```python
from build123d import *

# Parameters (mm, degrees)
SKETCH1_W           = 60
SKETCH1_H           = 50
BOSS_EXTRUDE1_DEPTH = 1
SKETCH2_R           = 0.25
CUT_EXTRUDE1_DEPTH  = 1.5
LPATTERN1_COUNT     = 3
LPATTERN1_PITCH     = 20
SKETCH3_R           = 0.25
CUT_EXTRUDE2_DEPTH  = 1.5
LPATTERN2_COUNT     = 3
LPATTERN2_PITCH     = 20
SKETCH4_R           = 0.5
CUT_EXTRUDE3_DEPTH  = 1.5
SKETCH5_R           = 0.25
CUT_EXTRUDE4_DEPTH  = 1.5
SKETCH6_R           = 0.2
CUT_EXTRUDE5_DEPTH  = 1.5
SKETCH7_R           = 0.25
CUT_EXTRUDE6_DEPTH  = 1.5
LPATTERN3_COUNT     = 7
LPATTERN3_PITCH     = 2.5
SKETCH8_R           = 0.25
CUT_EXTRUDE7_DEPTH  = 1.5
SKETCH9_R           = 0.875
CUT_EXTRUDE8_DEPTH  = 1.5
SKETCH10_R          = 0.5
CUT_EXTRUDE9_DEPTH  = 1.5
SKETCH11_R          = 0.25
CUT_EXTRUDE10_DEPTH = 1.5
SKETCH12_R          = 0.25
CUT_EXTRUDE11_DEPTH = 1.5


with BuildPart() as part:
    # Sketch1 → Boss-Extrude1 (new body)
    with BuildSketch(Plane(origin=(0, 0, 0), x_dir=(1, 0, 0), z_dir=(0, 1, 0))):
        with Locations((30, 25)):
            Rectangle(SKETCH1_W, SKETCH1_H)
    extrude(amount=BOSS_EXTRUDE1_DEPTH)

    # Sketch2 → Cut-Extrude1 (cut)
    with BuildSketch(Plane(origin=(0, 1, 0), x_dir=(1, 0, 0), z_dir=(0, 1, 0))):
        with Locations((10, 7)):
            Circle(SKETCH2_R)
    cut_extrude1 = extrude(amount=-CUT_EXTRUDE1_DEPTH, mode=Mode.SUBTRACT)

    # LPattern1: Cut-Extrude1 ×3
    with Locations(*[(i * LPATTERN1_PITCH, 0, 0) for i in range(1, LPATTERN1_COUNT)]):
        add(cut_extrude1, mode=Mode.SUBTRACT)

    # Sketch3 → Cut-Extrude2 (cut)
    with BuildSketch(Plane(origin=(0, 1, 0), x_dir=(1, 0, 0), z_dir=(0, 1, 0))):
        with Locations((10, 8.5)):
            Circle(SKETCH3_R)
    cut_extrude2 = extrude(amount=-CUT_EXTRUDE2_DEPTH, mode=Mode.SUBTRACT)

    # LPattern2: Cut-Extrude2 ×3
    with Locations(*[(i * LPATTERN2_PITCH, 0, 0) for i in range(1, LPATTERN2_COUNT)]):
        add(cut_extrude2, mode=Mode.SUBTRACT)

    # Sketch4 → Cut-Extrude3 (cut)
    with BuildSketch(Plane(origin=(0, 1, 0), x_dir=(1, 0, 0), z_dir=(0, 1, 0))):
        with Locations((2.5, 20)):
            Circle(SKETCH4_R)
        with Locations((2.5, 25.5)):
            Circle(SKETCH4_R)
    extrude(amount=-CUT_EXTRUDE3_DEPTH, mode=Mode.SUBTRACT)

    # Sketch5 → Cut-Extrude4 (cut)
    with BuildSketch(Plane(origin=(0, 1, 0), x_dir=(1, 0, 0), z_dir=(0, 1, 0))):
        with Locations((10, 20)):
            Circle(SKETCH5_R)
        with Locations((11.25, 22.5)):
            Circle(SKETCH5_R)
        with Locations((8.75, 22.5)):
            Circle(SKETCH5_R)
    extrude(amount=-CUT_EXTRUDE4_DEPTH, mode=Mode.SUBTRACT)

    # Sketch6 → Cut-Extrude5 (cut)
    with BuildSketch(Plane(origin=(0, 1, 0), x_dir=(1, 0, 0), z_dir=(0, 1, 0))):
        with Locations((16.25, 22.5)):
            Circle(SKETCH6_R)
        with Locations((16.25, 28)):
            Circle(SKETCH6_R)
    extrude(amount=-CUT_EXTRUDE5_DEPTH, mode=Mode.SUBTRACT)

    # Sketch7 → Cut-Extrude6 (cut)
    with BuildSketch(Plane(origin=(0, 1, 0), x_dir=(1, 0, 0), z_dir=(0, 1, 0))):
        with Locations((25.25, 28)):
            Circle(SKETCH7_R)
        with Locations((25.25, 20.5)):
            Circle(SKETCH7_R)
    cut_extrude6 = extrude(amount=-CUT_EXTRUDE6_DEPTH, mode=Mode.SUBTRACT)

    # LPattern3: Cut-Extrude6 ×7
    with Locations(*[(i * LPATTERN3_PITCH, 0, 0) for i in range(1, LPATTERN3_COUNT)]):
        add(cut_extrude6, mode=Mode.SUBTRACT)

    # Sketch8 → Cut-Extrude7 (cut)
    with BuildSketch(Plane(origin=(0, 1, 0), x_dir=(1, 0, 0), z_dir=(0, 1, 0))):
        with Locations((50, 35)):
            Circle(SKETCH8_R)
        with Locations((50, 36.5)):
            Circle(SKETCH8_R)
    extrude(amount=-CUT_EXTRUDE7_DEPTH, mode=Mode.SUBTRACT)

    # Sketch9 → Cut-Extrude8 (cut)
    with BuildSketch(Plane(origin=(0, 1, 0), x_dir=(1, 0, 0), z_dir=(0, 1, 0))):
        with Locations((56.5, 46.5)):
            Circle(SKETCH9_R)
        with Locations((3.5, 46.5)):
            Circle(SKETCH9_R)
    extrude(amount=-CUT_EXTRUDE8_DEPTH, mode=Mode.SUBTRACT)

    # Sketch10 → Cut-Extrude9 (cut)
    with BuildSketch(Plane(origin=(0, 1, 0), x_dir=(1, 0, 0), z_dir=(0, 1, 0))):
        with Locations((47, 47)):
            Circle(SKETCH10_R)
        with Locations((41, 47)):
            Circle(SKETCH10_R)
        with Locations((26, 47)):
            Circle(SKETCH10_R)
        with Locations((20, 47)):
            Circle(SKETCH10_R)
    extrude(amount=-CUT_EXTRUDE9_DEPTH, mode=Mode.SUBTRACT)

    # Sketch11 → Cut-Extrude10 (cut)
    with BuildSketch(Plane(origin=(0, 1, 0), x_dir=(1, 0, 0), z_dir=(0, 1, 0))):
        with Locations((47, 43)):
            Circle(SKETCH11_R)
        with Locations((34.5, 43)):
            Circle(SKETCH11_R)
        with Locations((26, 43)):
            Circle(SKETCH11_R)
        with Locations((13.5, 43)):
            Circle(SKETCH11_R)
    extrude(amount=-CUT_EXTRUDE10_DEPTH, mode=Mode.SUBTRACT)

    # Sketch12 → Cut-Extrude11 (cut)
    with BuildSketch(Plane(origin=(0, 1, 0), x_dir=(1, 0, 0), z_dir=(0, 1, 0))):
        with Locations((10, 36.5)):
            Circle(SKETCH12_R)
        with Locations((10, 35)):
            Circle(SKETCH12_R)
    extrude(amount=-CUT_EXTRUDE11_DEPTH, mode=Mode.SUBTRACT)


solid = part.part
```
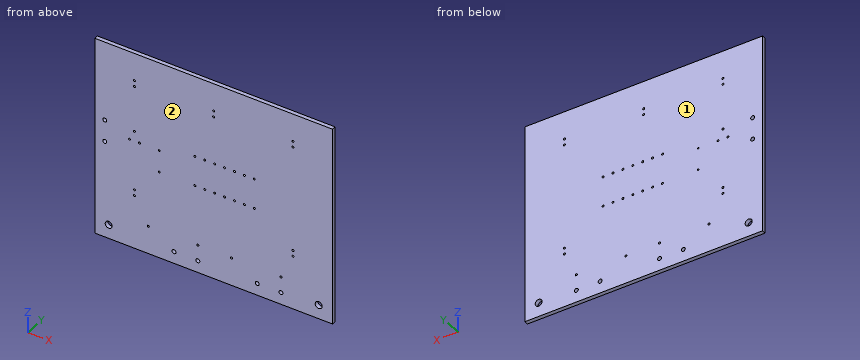
CAD build for the part. Positions are in the model's coordinates, mm. Face numbers are marked on the shaded views. Round coordinates to 2 decimals unless told otherwise and drop trailing zeros. Loops run counter-clockwise (first coordinate to the right, second up) from the corner with the lowest first, then second, coordinate; pieces in that order, holes last. Notation, with made-up numbers: M 80,38 L 105,38 A33 cw 105,71 Z; hole C 2.25,73 d2. An arc over 180 degrees is marked long. Return JSON: item names as keys, results as strings. Group by question number.
(1) Mould opens along Y. For the marked faces 1 and 2 say: +Y half, -Y half, draft (parallel to the pull), parting line (faces both ways), or undercut.
(2) Wall check: probe 1 along X at (y, z) = (0.35, -22.5); probe 2 along Z at (x, y) = (2.5, 0.7); probe 3 along Z at (x, y) = (37.75, 0.6). Give the ranges that are in metal, low to high. Write a range as [from, to].
(3) Saw through at A-A, the plane x = 56.5. List the corners of the cut face in (y, z) (3 decimals).
Answer list:
{
 "1": {"face 1": "+Y half", "face 2": "-Y half"},
 "2": {"probe 1": "[0, 8.5], [9, 11], [11.5, 16.05], [16.45, 60]", "probe 2": "[-50, -26], [-25, -20.5], [-19.5, 0]", "probe 3": "[-50, -28.25], [-27.75, -20.75], [-20.25, 0]"},
 "3": {"outline": "M 0,-50 L 1,-50 L 1,-47.375 L 0,-47.375 Z; M 0,-45.625 L 1,-45.625 L 1,0 L 0,0 Z"}
}
